Build history of the part. All positions in model axes, mm. Give positions to 0.01 mm unless a question says otherwise; leave off trailing zeros. Loops run counter-clockwise (first coordinate to the right, second up) from the corner with the lowest first, then second, coordinate; pieces in that order, holes last. Notation, with made-up numbers: M 55.5,3 L 104.5,3 A9 cw 104.5,18 Z; hole C 25.5,25.5 d9. An arc over 180 degrees is marked long. Answer as a JSON object with one key per item and string values. Group by question number.
1. Drill centre lines: line 1 along Z through (x, y) = (1.4, 0) (3 decimals); line 2 along Y through (x, z) = (2.25, 0.75); line 3 along Y through (x, z) = (3, 0.25). Where is each one in solid material? Low to high. Write a range as [from, to].
2. Slice it at D-D (x = 2.6). List the corners of the cut face in (y, z), then the cut area to 3 significant figures.
3. Slice it at A-A (y = 0). List the corners of the cut face in (x, z) (3 decimals).
4. Drop a flat-ended pin along its axis: pin 1 Ø1.5 at (x, y) = (4, -1) entering from +Z. Give the stop position or say it passes through.
5. Mould opens along Z. For faces 1 (the face through (3, 0, -2)), 2 (the face through (0, -2, 2)), 3 (the face through (0.987, -0.753, 3.392)) say: released by +Z, released by -Z, zero draft, split by the parting line, or undercut.
6. Slice it at C-C (x = 0.9). List the corners of the cut face in (y, z) (3 decimals).
Autodesk Inventor part; units mm, degrees
ref_plane "YZ Plane" through (0, 0, 0) normal (1, 0, 0) x (0, 1, 0)
ref_plane "XZ Plane" through (0, 0, 0) normal (0, 1, 0) x (-1, 0, 0)
ref_plane "XY Plane" through (0, 0, 0) normal (0, 0, 1) x (1, 0, 0)
sketch "Sketch_40" plane through (0, 0, 0) normal (0, 0, 1) x (1, 0, 0)
  line L0 (2.5, 0) -> (-2.5, 0)
  line L1 (0, 3.425) -> (0, 2.2)
  arc A0 (0, 2.2) -> (0.2, 2) centre (0.2, 2.2) ccw
  line L2 (0.2, 2) -> (4.8, 2)
  arc A1 (4.8, 2) -> (5, 2.2) centre (4.8, 2.2) ccw
  line L3 (5, 2.2) -> (5, 3.425)
  arc A2 (5, 3.425) -> (4.95, 3.475) centre (4.95, 3.425) ccw
  line L4 (4.95, 3.475) -> (3.3073, 3.475)
  arc A3 (1.6927, 3.475) -> (3.3073, 3.475) centre (2.5, 4.35) ccw
  line L5 (1.6927, 3.475) -> (0.05, 3.475)
  arc A4 (0.05, 3.475) -> (0, 3.425) centre (0.05, 3.425) ccw
revolve "Revolution1" add sketch "Sketch_40" angle 360 about axis through (2.5, 0, 0) along (1, 0, 0)
sketch "Sketch_42" plane through (0, 0, 0) normal (0, 0, 1) x (1, 0, 0)
  line L0 (2.5, 0) -> (-2.5, 0)
  line L1 (0, 7.35) -> (0, 3)
  line L2 (0, 3) -> (0.1, 3)
  arc A0 (0.1, 3) -> (0.3, 3.2) centre (0.1, 3.2) ccw
  line L3 (0.3, 3.2) -> (0.3, 7.15)
  line L4 (0.3, 7.15) -> (4.7, 7.15)
  line L5 (4.7, 7.15) -> (4.7, 3.2)
  arc A1 (4.7, 3.2) -> (4.9, 3) centre (4.9, 3.2) ccw
  line L6 (4.9, 3) -> (5, 3)
  line L7 (5, 3) -> (5, 7.35)
  line L8 (5, 7.35) -> (0, 7.35)
revolve "Revolution2" cut sketch "Sketch_42" angle 360 about axis through (2.5, 0, 0) along (1, 0, 0)
properties part number "SKF_W 624 R_PART1"
Established:
{
 "1": {"line 1": "z = [-3.475, -2], [2, 3.475]", "line 2": "y = [-3.1, -1.85], [1.85, 3.1]", "line 3": "y = [-3.26, -1.98], [1.98, 3.26]"},
 "2": {"outline": "C 0,0 d6.33; hole C 0,0 d4", "area": "18.9 mm^2"},
 "3": {"outline": "M 0,-3 L 0.1,-3 A0.2 cw 0.3,-3.2 L 0.3,-3.475 L 1.693,-3.475 A1.191 cw 3.307,-3.475 L 4.7,-3.475 L 4.7,-3.2 A0.2 cw 4.9,-3 L 5,-3 L 5,-2.2 A0.2 ccw 4.8,-2 L 0.2,-2 A0.2 ccw 0,-2.2 Z; M 0,2.2 A0.2 ccw 0.2,2 L 4.8,2 A0.2 ccw 5,2.2 L 5,3 L 4.9,3 A0.2 cw 4.7,3.2 L 4.7,3.475 L 3.307,3.475 A1.191 cw 1.693,3.475 L 0.3,3.475 L 0.3,3.2 A0.2 cw 0.1,3 L 0,3 Z"},
 "4": {"pin 1": "stops at z = 3.47"},
 "5": {"face 1": "undercut", "face 2": "zero draft", "face 3": "split by the parting line"},
 "6": {"outline": "C 0,0 d6.95; hole C 0,0 d4"}
}
